Geometry: final body of the model. Coordinates: model frame, mm. A direction names the side the tool comes from. Coordinates: 2 decimals unless noted, no trailing zeros. Write each loop counter-clockwise with the first axis right and the second up, starting at its lowest first coordinate (ties: lowest second). Pieces come first, ordered by that corner, then holes. Notation, with made-up numbers: (39, 6.25) - (51, 6.25) arc R14 cw to (51, 33.25) - close; hole circle Ø1 at (20, -14.75). An arc over 180 degrees is marked (long way). Answer as a JSON object with one key per item and string values. Group by question number.
Item 1: Line query: line 1 along X through (y, z) = (0, 0.1); line 2 along Y through (x, z) = (0, -0.45). Output: solid intervals per line, ascending. Write a range as from..to.
Item 2: Mould query, pull axis Y, two halves, no side actions, for faces 1 (the flat face through (0, 3.5, 1)), 2 (the cylindrical face through (2.86, -0.9, -0.49)), 3 (the flat face through (2, 1, -1)), 4 (the cylindrical face through (-3.16, -3.183, 5.246)). Classes: pulls with the +Y half, pulls with the -Y half, needs draft (parallel to the pull), parting line crosses it, or undercut.
Item 3: Section D-D on z = 1.75. Return loops of the section in (x, y), and give its area (4 significant figures).
Item 4: Section B-B on z = 4.5. Return loops of the section in (x, y), and give its area (3 significant figures).
Item 5: First-contact query: pin 1 Ø4 at (x, z) = (1, 4.5) entering from -Y; pin 2 Ø1.1 at (x, y) = (-3, -3) entering from -Z. Flat tips, straight axial feed; report the tip coordinate or a pass-through.
Item 6: Set-up query: faces 5 (the cylindrical face through (3.183, -3.16, 5.246)), 6 (the cylindrical face through (-0.31, 2.01, -0.21)), 7 (the flat face through (3.5, 0, 1)). Return all of +Z, -Z, +X, -X, +Y, -Y with unobstructed straight access to the full face (end or side cutting, diameter ignored); none if empty.
Item 7: Section C-C on y = -0.5. Return loops of the section in (x, z), and give its area (3 significant figures).
```python
from build123d import *

# Parameters (mm, degrees)
ESQUISSE1_W                        = 7
ESQUISSE1_H                        = 7
BOSS_EXTRU_1_DEPTH                 = 2
ESQUISSE2_R                        = 3
ESQUISSE2_R_2                      = 2.032039
BOSS_EXTRU_2_DEPTH                 = 1
ESQUISSE3_R                        = 0.75
BOSS_EXTRU_3_DEPTH                 = 3
BOSS_EXTRU_4_DEPTH                 = 1
CONG_1_R                           = 0.5
R_P_TITION_CIRCULAIRE2_COUNT       = 4
CONG_1_OF_R_P_TITION_CIRCULAIRE2_R = 0.5
ESQUISSE6_W                        = 3.5
ESQUISSE6_H                        = 3.5
ENL_V_MAT_EXTRU_1_DEPTH            = 1
ENL_V_START                        = -1
ESQUISSE7_R                        = 2.032039
ENL_V_MAT_EXTRU_2_DEPTH            = 1


with BuildPart() as part:
    # Esquisse1 → Boss.-Extru.1 (new body)
    with BuildSketch(Plane.XY):
        Rectangle(ESQUISSE1_W, ESQUISSE1_H)
    extrude(amount=BOSS_EXTRU_1_DEPTH)

    # Esquisse2 → Boss.-Extru.2 (add)
    with BuildSketch(Plane(origin=(0, 0, 0), x_dir=(-1, 0, 0), z_dir=(0, 0, -1))):
        with Locations(Location((0, 0, 0), (0, 0, 180))):
            Circle(ESQUISSE2_R)
        Circle(ESQUISSE2_R_2, mode=Mode.SUBTRACT)
    extrude(amount=BOSS_EXTRU_2_DEPTH)

    # Esquisse3 → Boss.-Extru.3 (add)
    with BuildSketch(Plane(origin=(-0.00837, -0.443983, 2), x_dir=(1, 0, 0), z_dir=(0, 0, 1))):
        with Locations((-2.49163, 2.943983)):
            Circle(ESQUISSE3_R)
    boss_extru_3 = extrude(amount=BOSS_EXTRU_3_DEPTH)

    # Esquisse5 → Boss.-Extru.4 (add)
    with BuildSketch(Plane.XY.offset(5)):
        with BuildLine():
            Line((-3.03033, 1.96967), (-3.171751, 2.111091))
            ThreePointArc((-3.171751, 2.111091), (-3.171751, 3.171751), (-2.111091, 3.171751))
            Line((-2.111091, 3.171751), (-1.96967, 3.03033))
            ThreePointArc((-1.96967, 3.03033), (-1.96967, 1.96967), (-3.03033, 1.96967))
        make_face()
    boss_extru_4 = extrude(amount=BOSS_EXTRU_4_DEPTH)

    # Congé1
    cong_1_edges = [part.edges().sort_by_distance(p)[0] for p in [
        (-1.96967, 1.96967, 6),
        (-2.040381, 3.101041, 6),
        (-3.171751, 3.171751, 6),
        (-3.101041, 2.040381, 6),
    ]]
    fillet(cong_1_edges, radius=CONG_1_R)

    # Répétition circulaire2: Boss.-Extru.3, Boss.-Extru.4 ×4 about axis
    r_p_tition_circulaire2_axis = Axis((0, 0, 0), (0, 0, 1))
    add([boss_extru_3.rotate(r_p_tition_circulaire2_axis, i * 360 / R_P_TITION_CIRCULAIRE2_COUNT) for i in range(1, R_P_TITION_CIRCULAIRE2_COUNT)])
    add([boss_extru_4.rotate(r_p_tition_circulaire2_axis, i * 360 / R_P_TITION_CIRCULAIRE2_COUNT) for i in range(1, R_P_TITION_CIRCULAIRE2_COUNT)])

    # Congé1 of Répétition circulaire2
    cong_1_of_r_p_tition_circulaire2_edges = [part.edges().sort_by_distance(p)[0] for p in [
        (-1.96967, -1.96967, 6),
        (-3.101041, -2.040381, 6),
        (-3.171751, -3.171751, 6),
        (-2.040381, -3.101041, 6),
        (1.96967, -1.96967, 6),
        (2.040381, -3.101041, 6),
        (3.171751, -3.171751, 6),
        (3.101041, -2.040381, 6),
        (1.96967, 1.96967, 6),
        (3.101041, 2.040381, 6),
        (3.171751, 3.171751, 6),
        (2.040381, 3.101041, 6),
    ]]
    fillet(cong_1_of_r_p_tition_circulaire2_edges, radius=CONG_1_OF_R_P_TITION_CIRCULAIRE2_R)

    # Esquisse6 → Enlèv. mat.-Extru.1 (cut)
    with BuildSketch(Plane.XY.offset(2)):
        Rectangle(ESQUISSE6_W, ESQUISSE6_H)
    extrude(amount=-ENL_V_MAT_EXTRU_1_DEPTH, mode=Mode.SUBTRACT)

    # Esquisse7 → Enlèv. mat.-Extru.2 (cut)
    with BuildSketch(Plane(origin=(0, 0, 0), x_dir=(-1, 0, 0), z_dir=(0, 0, -1)).offset(ENL_V_START)):
        with Locations(Location((0, 0, 0), (0, 0, 149.452052))):
            Circle(ESQUISSE7_R)
    extrude(amount=ENL_V_MAT_EXTRU_2_DEPTH, mode=Mode.SUBTRACT)


solid = part.part
```
Checks:
{
 "1": {"line 1": "-3.5..-2.03, 2.03..3.5", "line 2": "-3..-2.03, 2.03..3"},
 "2": {"face 1": "pulls with the +Y half", "face 2": "parting line crosses it", "face 3": "needs draft", "face 4": "undercut"},
 "3": {"outline": "(-3.5, -3.5) - (3.5, -3.5) - (3.5, 3.5) - (-3.5, 3.5) - close; hole (-1.75, -1.75) - (1.75, -1.75) - (1.75, 1.75) - (-1.75, 1.75) - close", "area": "36.75 mm^2"},
 "4": {"outline": "circle Ø1.5 at (-2.5, -2.5); circle Ø1.5 at (-2.5, 2.5); circle Ø1.5 at (2.5, -2.5); circle Ø1.5 at (2.5, 2.5)", "area": "7.07 mm^2"},
 "5": {"pin 1": "y = -3.39", "pin 2": "z = 0"},
 "6": {"face 5": "+Z", "face 6": "-Z", "face 7": "+Z, -Z, +X, +Y, -Y"},
 "7": {"outline": "(-3.5, 0) - (-2.96, 0) - (-2.96, -1) - (-1.97, -1) - (-1.97, 1) - (-1.75, 1) - (-1.75, 2) - (-3.5, 2) - close; (1.75, 1) - (1.97, 1) - (1.97, -1) - (2.96, -1) - (2.96, 0) - (3.5, 0) - (3.5, 2) - (1.75, 2) - close", "area": "8.54 mm^2"}
}
